from build123d import *

# Parameters (mm, degrees)
SKETCH1_R               = 25.795
SKETCH1_R_2             = 18.885
BOSS_EXTRUDE1_DEPTH     = 67.2
SKETCH2_R               = 21.795
SKETCH2_R_2             = 21.195
CUT_EXTRUDE2_DEPTH      = 10.73
CUT_EXTRUDE3_DEPTH      = 77.463089462
CUT_EXTRUDE3_DEPTH_BACK = 77.463089462
SKETCH3_R               = 21.195
SKETCH3_R_2             = 18.885
SKETCH4_R               = 26.36
BOSS_EXTRUDE2_DEPTH     = 15.9
SKETCH5_R               = 26.415
BOSS_EXTRUDE3_DEPTH     = 57.51
CUT_EXTRUDE6_DEPTH      = 83.368273929
CUT_EXTRUDE6_DEPTH_BACK = 83.368273929
SKETCH10_R              = 19.607658562


with BuildPart() as part:
    # Sketch1 → Boss-Extrude1 (new body)
    with BuildSketch(Plane.XY):
        Circle(SKETCH1_R)
        Circle(SKETCH1_R_2, mode=Mode.SUBTRACT)
    extrude(amount=BOSS_EXTRUDE1_DEPTH)

    # Sketch2 → Cut-Extrude2 (cut)
    with BuildSketch(Plane(origin=(0, 0, 0), x_dir=(-1, 0, 0), z_dir=(0, 0, -1))):
        Circle(SKETCH2_R)
        Circle(SKETCH2_R_2, mode=Mode.SUBTRACT)
    extrude(amount=-CUT_EXTRUDE2_DEPTH, mode=Mode.SUBTRACT)

    # Sketch3 → Cut-Extrude3 (cut, two sides: drawn at the far end of the back side and taken through both)
    with BuildSketch(Plane(origin=(0, 0, 0), x_dir=(-1, 0, 0), z_dir=(0, 0, -1)).offset(-CUT_EXTRUDE3_DEPTH_BACK)):
        Circle(SKETCH3_R)
        Circle(SKETCH3_R_2, mode=Mode.SUBTRACT)
    extrude(amount=CUT_EXTRUDE3_DEPTH + CUT_EXTRUDE3_DEPTH_BACK, mode=Mode.SUBTRACT)

    # Sketch4 → Boss-Extrude2 (add)
    with BuildSketch(Plane.XY.offset(67.2)):
        Circle(SKETCH4_R)
    extrude(amount=-BOSS_EXTRUDE2_DEPTH)

    # Sketch5 → Boss-Extrude3 (add)
    with BuildSketch(Plane.XY.offset(67.2)):
        Circle(SKETCH5_R)
    extrude(amount=BOSS_EXTRUDE3_DEPTH)

    # Sketch10 → Cut-Extrude6 (cut, two sides: drawn at the far end of the back side and taken through both)
    with BuildSketch(Plane(origin=(0, 0, 51.3), x_dir=(-1, 0, 0), z_dir=(0, 0, -1)).offset(-CUT_EXTRUDE6_DEPTH_BACK)):
        Circle(SKETCH10_R)
    extrude(amount=CUT_EXTRUDE6_DEPTH + CUT_EXTRUDE6_DEPTH_BACK, mode=Mode.SUBTRACT)


solid = part.part
The listing builds one solid part. Answer for the finished solid, in the listing's coordinates (mm). A direction names the side the tool comes from. Coordinates: 2 decimals unless noted, no trailing zeros. Write each loop counter-clockwise with the first axis right and the second up, starting at its lowest first coordinate (ties: lowest second). Pieces come first, ordered by that corner, then holes. Notation, with made-up numbers: M 46.25,21.25 L 50.25,21.25 A21 cw 50.25,40.25 Z; hole C -24,-19 d7. An arc over 180 degrees is marked long. Use one line per item in the form item = value.
Item 1: Find section A-A, the plane x = 0. Give the vertices of the cut face in (y, z) (3 decimals), plus the area to 3 significant figures.
Model answer:
outline = M -26.415,67.2 L -26.36,67.2 L -26.36,51.3 L -25.795,51.3 L -25.795,0 L -21.795,0 L -21.795,10.73 L -21.195,10.73 L -21.195,51.3 L -19.608,51.3 L -19.608,124.71 L -26.415,124.71 Z; M 19.608,51.3 L 21.195,51.3 L 21.195,10.73 L 21.795,10.73 L 21.795,0 L 25.795,0 L 25.795,51.3 L 26.36,51.3 L 26.36,67.2 L 26.415,67.2 L 26.415,124.71 L 19.608,124.71 Z
area = 1,460 mm2
Item 2: Find section C-C, the plane z = 64. Give the vertices of the cut face in (x, y).
Model answer:
outline = C 0,0 d52.72; hole C 0,0 d39.22
Item 3: For faces 4 (the face through (6, -19, 51.3)), 5 (the face through (-5.726, -25.787, 95.552)), determine the directions among +Z, -Z, +X, -X, +Y, -Y from which every point of the face is accessible in a straight line to the end or side of a thin tool.
Model answer:
face_4 = -Z
face_5 = +Z, -Z
Item 4: The mould has two halves that part along Y. Classify faces 1 (the face through (-12, 19, 0)), 2 (the face through (-18.7, 5.9, 88.5)), 3 (the face through (25.14, 7.92, 59.36)): released by +Y, released by -Y, zero draft, split by the parting line, or undercut.
Model answer:
face_1 = zero draft
face_2 = undercut
face_3 = split by the parting line
Item 5: Given P1, Ø12, axis at x = -6, z = 39, coming from the -Y side (3 decimals); P2, Ø2, axis at x = -8.5, z = 111.5, coming from the +Y side; P3, Ø12, axis at y = 20.5, z = 44.5, coming from the -X side, each flat-ended and moving along its own axis, determine where each tip first touches the part or whether it passes through.
Model answer:
P1 = -25.795
P2 = 25.33
P3 = -21.33
Item 6: Find the intervals of material crossed by probe 1 along Y at (x, z) = (0, 103) (3 decimals); probe 2 along Y at (x, z) = (0, 40) (3 decimals), in increasing order.
Model answer:
probe_1 = -26.415 to -19.608, 19.608 to 26.415
probe_2 = -25.795 to -21.195, 21.195 to 25.795
Item 7: Find section D-D, the plane z = 29. Give the vertices of the cut face in (x, y) (3 decimals), plus the area to 3 significant figures.
Model answer:
outline = C 0,0 d51.59; hole C 0,0 d42.39
area = 679 mm2
